from build123d import *

# Parameters (mm, degrees)
SKETCH1_R           = 3
BOSS_EXTRUDE1_DEPTH = 10
SKETCH2_R           = 1.75
CUT_EXTRUDE1_DEPTH  = 0.5
BOSS_EXTRUDE2_START = 0.1
SKETCH3_R           = 1.75
BOSS_EXTRUDE2_DEPTH = 0.1


with BuildPart() as part:
    # Sketch1 → Boss-Extrude1 (new body)
    with BuildSketch(Plane.XY):
        Circle(SKETCH1_R)
    extrude(amount=BOSS_EXTRUDE1_DEPTH)

    # Sketch2 → Cut-Extrude1 (cut)
    with BuildSketch(Plane.XY):
        Circle(SKETCH2_R)
    extrude(amount=CUT_EXTRUDE1_DEPTH, mode=Mode.SUBTRACT)

    # Sketch3 → Boss-Extrude2 (add)
    with BuildSketch(Plane(origin=(0, 0, 0.5), x_dir=(-1, 0, 0), z_dir=(0, 0, -1)).offset(BOSS_EXTRUDE2_START)):
        Circle(SKETCH3_R)
    extrude(amount=-BOSS_EXTRUDE2_DEPTH)


solid = part.part
Here's how the part is built. I have some questions about the finished solid (model axes, mm). A direction names the side the tool comes from. Give positions to 0.01 mm unless a question says otherwise; leave off trailing zeros. Write each loop counter-clockwise with the first axis right and the second up, starting at its lowest first coordinate (ties: lowest second). Pieces come first, ordered by that corner, then holes. Notation, with made-up numbers: (-26.5, -19) -> (-11.5, -19) arc R15 cw to (-11.5, -5) -> close; hole circle Ø10 at (89.5, 48.25). An arc over 180 degrees is marked (long way). Use one line per item in the form item = value. Start each with the question number.
1. Imagine slicing it at C-C on z = 6. List the corners of the cut face in (x, y) for me, plus the area to 3 significant figures.
2. Will these pins go through, and if not, where does the flat tip stop? pin 1 Ø1.5 at (y, z) = (2.5, 6) entering from -X; pin 2 Ø2 at (y, z) = (2, 9) entering from +X; pin 3 Ø1 at (y, z) = (-1.5, 2) entering from -X.
3. Imagine slicing it at A-A on x = 0. List the corners of the cut face in (y, z) for me.
4. Thinking about a two-plate mould opening in Y: for faces 3 (the face through (-3, 0, 5)), 4 (the face through (0, -2, 0)), 5 (the face through (1.617, -0.67, 0.197)), which applies, +Y half, -Y half, draft (parallel to the pull), parting line (faces both ways), or undercut?
5. Imagine slicing it at D-D on y = -2.35. List the corners of the cut face in (x, z) for me, plus the area to 3 significant figures.
6. On a 3-axis mill with a long thin cutter (end or side, diameter ignored), from which of +Z, -Z, +X, -X, +Y, -Y can I reach the whole of each face in a straight line? I mean faces 1 (the face through (0, 0, 0.4)), 2 (the face through (0, 0, 10)). Say none if no direction works.
7. If I drill on L1, parallel to Y at x = 0, z = 0.25; L2, parallel to Z at x = -0.85, y = 1.05; L3, parallel to Y at x = 2.4, z = 3.25, over which ranges is the centre line in solid material (lowest first)?
Entries:
q1.outline = circle Ø6 at (0, 0)
q1.area = 28.3 mm²
q2.pin_1 = -2.44
q2.pin_2 = 2.83
q2.pin_3 = -2.83
q3.outline = (-3, 0) -> (-1.75, 0) -> (-1.75, 0.4) -> (1.75, 0.4) -> (1.75, 0) -> (3, 0) -> (3, 10) -> (-3, 10) -> close
q4.face_3 = parting line
q4.face_4 = draft
q4.face_5 = undercut
q5.outline = (-1.86, 0) -> (1.86, 0) -> (1.86, 10) -> (-1.86, 10) -> close
q5.area = 37.3 mm²
q6.face_1 = -Z
q6.face_2 = +Z, +X, -X, +Y, -Y
q7.L1 = -3 to -1.75, 1.75 to 3
q7.L2 = 0.4 to 10
q7.L3 = -1.8 to 1.8
